Work out the finished part from the listing and answer in its coordinate system (mm). Coordinates: 2 decimals unless noted, no trailing zeros. Order: outer loops, then holes, each group sorted by start corner. A loop starts at its lowest first (then second) coordinate and runs counter-clockwise, first axis right, second up.
1. The part is cut by section B-B, the plane x = -8.75. Give the vertices of the cut face in (y, z).
2. Find the intervals of material crossed by probe 1 along Z at (x, y) = (-8.75, 1.8); probe 2 along X at (y, z) = (0.65, 27); probe 3 along X at (y, z) = (1.65, -18.5), in increasing order.
3. The part is cut by section A-A, the plane z = 27. Give the vertices of the cut face in (x, y).
4. The part is cut by section C-C, the plane z = 0. Give the vertices of the cut face in (x, y).
5. Determine the mould class of faces 1 (the flat face through (0, 1, -30)), 2 (the flat face through (17.5, 1, 0)), 3 (the flat face through (0, 1, 30)), 4 (the cylindrical face through (0.358, 1.479, -21.227)) for opening direction Z: +Z half, -Z half, draft (parallel to the pull), parting line (faces both ways), or undercut.
6. The part is cut by section D-D, the plane y = 1.1. Give the vertices of the cut face in (x, z).
```python
from build123d import *

# Parameters (mm, degrees)
SKETCH_1_W          = 35
SKETCH_1_H          = 60
EXTRUDE_1_DEPTH     = 3
HOLE_WIZARD_1_D     = 3.5
HOLE_WIZARD_2_D     = 5.5
SKETCH_8_R          = 4.5
CUT_EXTRUDE_1_DEPTH = 3


with BuildPart() as part:
    # 草图1 → 凸台-拉伸1 (new body)
    with BuildSketch(Plane(origin=(0, 0, 0), x_dir=(1, 0, 0), z_dir=(0, 1, 0))):
        Rectangle(SKETCH_1_W, SKETCH_1_H)
    extrude(amount=EXTRUDE_1_DEPTH)

    # 孔1 (through all)
    with Locations(Plane(origin=(0, 3, 0), x_dir=(1, 0, 0), z_dir=(0, 1, 0))):
        with Locations((-8.75, 27), (8.75, 27), (8.75, -27), (-8.75, -27)):
            Hole(HOLE_WIZARD_1_D / 2)

    # 孔2 (through all)
    with Locations(Plane(origin=(0, 3, 0), x_dir=(1, 0, 0), z_dir=(0, 1, 0))):
        with Locations((0, 18.5), (0, -18.5)):
            Hole(HOLE_WIZARD_2_D / 2)

    # 草图8 → 切除-拉伸1 (cut)
    with BuildSketch(Plane(origin=(0, 3, 0), x_dir=(1, 0, 0), z_dir=(0, 1, 0))):
        with Locations(Location((0, 0, 0), (0, 0, 270))):
            Circle(SKETCH_8_R)
    extrude(amount=-CUT_EXTRUDE_1_DEPTH, mode=Mode.SUBTRACT)


solid = part.part
```
Geometry says:
1. outline: (0, -30) - (3, -30) - (3, -28.75) - (0, -28.75) - close; (0, -25.25) - (3, -25.25) - (3, 25.25) - (0, 25.25) - close; (0, 28.75) - (3, 28.75) - (3, 30) - (0, 30) - close
2. probe 1: z = -30 to -28.75, -25.25 to 25.25, 28.75 to 30
2. probe 2: x = -17.5 to -10.5, -7 to 7, 10.5 to 17.5
2. probe 3: x = -17.5 to -2.75, 2.75 to 17.5
3. outline: (-17.5, 0) - (-10.5, 0) - (-10.5, 3) - (-17.5, 3) - close; (-7, 0) - (7, 0) - (7, 3) - (-7, 3) - close; (10.5, 0) - (17.5, 0) - (17.5, 3) - (10.5, 3) - close
4. outline: (-17.5, 0) - (-4.5, 0) - (-4.5, 3) - (-17.5, 3) - close; (4.5, 0) - (17.5, 0) - (17.5, 3) - (4.5, 3) - close
5. face 1: -Z half
5. face 2: draft
5. face 3: +Z half
5. face 4: undercut
6. outline: (-17.5, -30) - (17.5, -30) - (17.5, 30) - (-17.5, 30) - close; hole circle Ø3.5 at (-8.75, -27); hole circle Ø3.5 at (-8.75, 27); hole circle Ø9 at (0, 0); hole circle Ø5.5 at (0, -18.5); hole circle Ø5.5 at (0, 18.5); hole circle Ø3.5 at (8.75, -27); hole circle Ø3.5 at (8.75, 27)
